Read the model definition and answer for the solid it produces. Units are mm, in the model's axes. A direction names the side the tool comes from. Coordinates: 2 decimals unless noted, no trailing zeros. Loops run counter-clockwise (first coordinate to the right, second up) from the corner with the lowest first, then second, coordinate; pieces in that order, holes last. Notation, with made-up numbers: M -15.5,63.5 L -8.5,63.5 A30 cw -8.5,94.5 Z; hole C 17.5,64 d3. An arc over 180 degrees is marked long. Use one line per item in the form item = value. Start each with the question number.
1. A tool of negligible diameter and unlimited length cuts with its end or side. For faces 5 (the cylindrical face through (-21.97, 14.32, 0.47)), 6 (the cylindrical face through (17.75, 2.03, -3.03)), 7 (the flat face through (-18.35, 8, 0)), 8 (the flat face through (-8, 3, -3.6)), 9 (the flat face through (-21, 12.3, 0)), from which of +Z, -Z, +X, -X, +Y, -Y can it reach the whole face along a straight path? Write none if from no direction.
2. Flat-ended cylindrical pins translate along their axes: pin 1 (3.5 mm diameter, centred on x = -1, z = 1.5, fed in from +Y); pin 2 (6 mm diameter, centred on x = -17.5, y = 9.5, fed in from -Z); pin 3 (1 mm diameter, centred on y = 6, z = -1.5, fed in from -X); pin 4 (2 mm diameter, centred on y = 7.5, z = 0.5, fed in from +X). Find the tip coordinate at first contact, or state that the pin passes through.
3. The part is cut by section C-C (y = 11.5). Give the vertices of the cut face in (x, z).
4. For a pull along Y with two mould halves and no side action, classify faces 1 (the flat face through (-2, 0, 0)), 2 (the flat face through (-24.35, 13, 0)), 3 (the cylindrical face through (-21.39, 10.77, -2.55)), 4 (the flat face through (0, 4, 0)) as released by +Y, released by -Y, zero draft, split by the parting line, or undercut.
5. The part is cut by section D-D (y = 8.25). Give the vertices of the cut face in (x, z).
6. The part is cut by section A-A (x = 15.25). Give the vertices of the cut face in (y, z), plus the area to 3 significant figures.
7. The part is cut by section B-B (z = 0). Give the vertices of the cut face in (x, y), plus the area to 3 significant figures.
8. Find the intervals of material crossed by probe 1 along X at (y, z) = (2.95, 0); probe 2 along Y at (x, z) = (14, 0); probe 3 along X at (y, z) = (7.25, 2.5), in increasing order. Write a range as [from, to].
from build123d import *

# Parameters (mm, degrees)
SKETCH1_W           = 36.7
SKETCH1_H           = 7.2
SKETCH1_R           = 1.1
BOSS_EXTRUDE1_DEPTH = 4
SKETCH2_W           = 4
SKETCH2_H           = 7.2
BOSS_EXTRUDE2_DEPTH = 10.75
SKETCH3_R           = 3.6
BOSS_EXTRUDE3_DEPTH = 6
FILLET1_R           = 2
CUT_EXTRUDE1_DEPTH  = 6


with BuildPart() as part:
    # Sketch1 → Boss-Extrude1 (new body)
    with BuildSketch(Plane(origin=(0, 0, 0), x_dir=(1, 0, 0), z_dir=(0, 1, 0))):
        Rectangle(SKETCH1_W, SKETCH1_H)
        with Locations(Location((15.25, 0, 0), (0, 0, 270))):
            Circle(SKETCH1_R, mode=Mode.SUBTRACT)
        with Locations(Location((-15.25, 0, 0), (0, 0, 270))):
            Circle(SKETCH1_R, mode=Mode.SUBTRACT)
    extrude(amount=BOSS_EXTRUDE1_DEPTH)

    # Sketch2 → Boss-Extrude2 (add)
    with BuildSketch(Plane.XZ):
        with Locations((-20.35, 0)):
            Rectangle(SKETCH2_W, SKETCH2_H)
    extrude(amount=-BOSS_EXTRUDE2_DEPTH)

    # Sketch3 → Boss-Extrude3 (add)
    with BuildSketch(Plane(origin=(-18.35, 0, 0), x_dir=(0, 0, -1), z_dir=(1, 0, 0))):
        with Locations((0, 10.75)):
            Circle(SKETCH3_R)
    extrude(amount=-BOSS_EXTRUDE3_DEPTH)

    # Fillet1
    fillet1_edges = [part.edges().sort_by_distance(p)[0] for p in [
        (18.35, 2, -3.6),
        (18.35, 2, 3.6),
    ]]
    fillet(fillet1_edges, radius=FILLET1_R)

    # Sketch4 → Cut-Extrude1 (cut)
    with BuildSketch(Plane.ZY.offset(24.35)):
        with BuildLine():
            Line((-2.024845673, 9.2), (0, 9.2))
            Line((0, 9.2), (0, 12.3))
            Line((0, 12.3), (-2.024845673, 12.3))
            ThreePointArc((-2.024845673, 12.3), (-2.55, 10.75), (-2.024845673, 9.2))
        make_face()
        with BuildLine():
            Line((0, 12.3), (0, 9.2))
            Line((0, 9.2), (2.024845673, 9.2))
            ThreePointArc((2.024845673, 9.2), (2.415145593, 9.93172635), (2.55, 10.75))
            ThreePointArc((2.55, 10.75), (2.415145593, 11.56827365), (2.024845673, 12.3))
            Line((2.024845673, 12.3), (0, 12.3))
        make_face()
    extrude(amount=-CUT_EXTRUDE1_DEPTH, mode=Mode.SUBTRACT)


solid = part.part
Computed values:
q1.face_5 = -X
q1.face_6 = -Z, +X, +Y, -Y
q1.face_7 = +Z, -Z, +X, +Y
q1.face_8 = -Z, +X, -X, +Y, -Y
q1.face_9 = +X, -X
q2.pin_1 = 4
q2.pin_2 = -3.6
q2.pin_3 = -22.35
q2.pin_4 = -18.35
q3.outline = M -24.35,-3.52 L -18.35,-3.52 L -18.35,-2.44 L -24.35,-2.44 Z; M -24.35,2.44 L -18.35,2.44 L -18.35,3.52 L -24.35,3.52 Z
q4.face_1 = released by -Y
q4.face_2 = zero draft
q4.face_3 = undercut
q4.face_4 = released by +Y
q5.outline = M -24.35,-2.59 L -22.35,-2.59 L -22.35,-3.6 L -18.35,-3.6 L -18.35,3.6 L -22.35,3.6 L -22.35,2.59 L -24.35,2.59 Z
q6.outline = M 0,-3.6 L 4,-3.6 L 4,-1.1 L 0,-1.1 Z; M 0,1.1 L 4,1.1 L 4,3.6 L 0,3.6 Z
q6.area = 20.0 mm²
q7.outline = M -24.35,7.15 L -22.35,7.15 L -22.35,0 L -16.35,0 L -16.35,4 L -18.35,4 L -18.35,9.2 L -24.35,9.2 Z; M -24.35,12.3 L -18.35,12.3 L -18.35,14.35 L -24.35,14.35 Z; M -14.15,0 L 14.15,0 L 14.15,4 L -14.15,4 Z; M 16.35,0 L 18.35,0 L 18.35,4 L 16.35,4 Z
q7.area = 182 mm²
q8.probe_1 = [-22.35, -16.35], [-14.15, 14.15], [16.35, 18.35]
q8.probe_2 = [0, 4]
q8.probe_3 = [-22.35, -18.35]
